Autodesk Inventor part; units mm, degrees
ref_plane "YZ Plane" through (0, 0, 0) normal (1, 0, 0) x (0, 1, 0)
ref_plane "XZ Plane" through (0, 0, 0) normal (0, 1, 0) x (-1, 0, 0)
ref_plane "XY Plane" through (0, 0, 0) normal (0, 0, 1) x (1, 0, 0)
sketch "Sketch2" plane through (0, 0, 0) normal (0, 0, 1) x (1, 0, 0)
  circle A0 centre (0, 0) radius 7
  dimension "d0" = 14
extrude "Extrusion1" add sketch "Sketch2" along normal blind 2
fillet "Fillet2" radius 0.5 1 edges at (-7, 0, 0)
hole "Hole1" at (0, 0, 0) direction (0, 0, 1) diameter 4.5 end through all
properties part number "P020" material "Aluminium"
Read the model definition and answer for the solid it produces. Units are mm, in the model's axes. Give positions to 0.01 mm unless a question says otherwise; leave off trailing zeros. Write each loop counter-clockwise with the first axis right and the second up, starting at its lowest first coordinate (ties: lowest second). Pieces come first, ordered by that corner, then holes. Notation, with made-up numbers: (-39.75, 30.25) - (-3.75, 30.25) arc R15 cw to (-3.75, 50.25) - close; hole circle Ø2 at (-7.5, 52.5). An arc over 180 degrees is marked (long way). Return JSON: item names as keys, results as strings.
Q1. Consider line 1 along Y through (x, z) = (0, 1.4); line 2 along X through (y, z) = (-2, 1.35); line 3 along X through (y, z) = (1.75, 1.65). Determine where each line is inside the solid, lowest interval first. Write a range as [from, to].
Reply:
{"line 1": "[-7, -2.25], [2.25, 7]", "line 2": "[-6.71, -1.03], [1.03, 6.71]", "line 3": "[-6.78, -1.41], [1.41, 6.78]"}
Q2. A cutting plane is placed at C-C, the plane z = 1.6. Determine the outline of the cut face in (x, y).
Reply:
{"outline": "circle Ø14 at (0, 0); hole circle Ø4.5 at (0, 0)"}
Q3. For a pull along Y with two mould halves and no side action, classify faces 1 (the face through (-2.23, -0.29, 1.01)), 2 (the face through (6.466, 2.681, 1.24)), 3 (the face through (3, 0, 0)) as released by +Y, released by -Y, zero draft, split by the parting line, or undercut.
Reply:
{"face 1": "undercut", "face 2": "split by the parting line", "face 3": "zero draft"}
Q4. A cutting plane is placed at A-A, the plane x = 0. Determine the outline of the cut face in (y, z).
Reply:
{"outline": "(-7, 0.5) arc R0.5 ccw to (-6.5, 0) - (-2.25, 0) - (-2.25, 2) - (-7, 2) - close; (2.25, 0) - (6.5, 0) arc R0.5 ccw to (7, 0.5) - (7, 2) - (2.25, 2) - close"}
Q5. Given P1, Ø1, axis at x = -2, z = 1, coming from the +Y side, flat-ended and moving along its own axis, determine where the tip first touches the part or whether it passes through.
Reply:
{"P1": "y = 6.84"}
